Can you work these out from the drawing? Everything is in mm from the part's minimum corner. Coordinates: 2 decimals unless noted, no trailing zeros. Write each loop counter-clockwise with the first axis right and the second up, starting at its lowest first coordinate (ties: lowest second). Pieces come first, ordered by that corner, then holes.
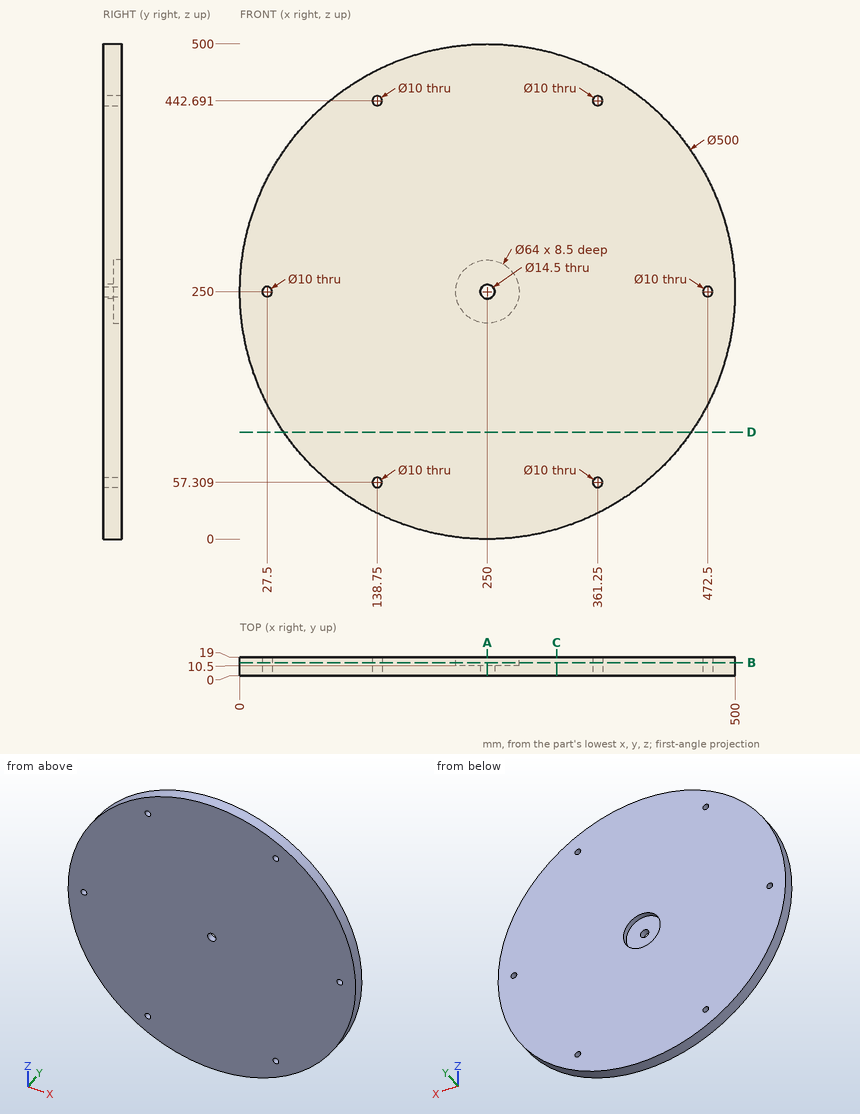
1. I want a section at A-A (x = 250). List the corners of the cut face in (y, z) for me, then the cut area to 3 significant figures.
2. I want a section at D-D (z = 108). List the corners of the cut face in (x, y) for me, then the cut area to 3 significant figures.
3. I want a section at C-C (x = 320). List the corners of the cut face in (y, z) for me.
4. If I drill on line 1 (X direction, y = 6.5, z = 250); line 2 (X direction, y = 15.25, z = 250); line 3 (Z direction, x = 27.5, y = 7.25), over which ranges is the centre line in solid material (lowest first)?
5. For pin 1 Ø6 at (x, z) = (361.25, 57.31) entering from -Y; pin 2 Ø4 at (x, y) = (64.5, 16) entering from -Z; pin 3 Ø4 at (x, y) = (150.5, 12) entering from +Z; pin 4 Ø5 at (y, z) = (16.5, 298.5) entering from +X, each with a flat end and sliding along its axis, tell me the tip position at first contact or that it passes through.
6. I want a section at B-B (y = 13.5). List the corners of the cut face in (x, z) for me, then the cut area to 3 significant figures.
Response values:
1. outline: (0, 0) - (19, 0) - (19, 218) - (10.5, 218) - (10.5, 242.75) - (0, 242.75) - close; (0, 257.25) - (10.5, 257.25) - (10.5, 282) - (19, 282) - (19, 500) - (0, 500) - close
1. area: 8,800 mm2
2. outline: (44.24, 0) - (455.76, 0) - (455.76, 19) - (44.24, 19) - close
2. area: 7,820 mm2
3. outline: (0, 10) - (19, 10) - (19, 490) - (0, 490) - close
4. line 1: x = 0 to 22.5, 32.5 to 242.75, 257.25 to 467.5, 477.5 to 500
4. line 2: x = 0 to 22.5, 32.5 to 218, 282 to 467.5, 477.5 to 500
4. line 3: z = 136.01 to 245, 255 to 363.99
5. pin 1: passes through
5. pin 2: stops at z = 80.21
5. pin 3: stops at z = 480.2
5. pin 4: stops at x = 495.73
6. outline: circle Ø500 at (250, 250); hole circle Ø10 at (27.5, 250); hole circle Ø10 at (138.75, 57.31); hole circle Ø10 at (138.75, 442.69); hole circle Ø64 at (250, 250); hole circle Ø10 at (361.25, 57.31); hole circle Ø10 at (361.25, 442.69); hole circle Ø10 at (472.5, 250)
6. area: 193,000 mm2
